from build123d import *

# Parameters (mm, degrees)
BOSS_EXTRUDE1_DEPTH = 6.35
SKETCH2_W           = 20
SKETCH2_H           = 6.35
CUT_EXTRUDE1_DEPTH  = 172.94569637
SKETCH4_W           = 6.35
SKETCH4_H           = 15
CUT_EXTRUDE2_DEPTH  = 172.94569637
FILLET1_R           = 2


with BuildPart() as part:
    # Sketch1 → Boss-Extrude1 (new body)
    with BuildSketch(Plane(origin=(0, 0, 0), x_dir=(1, 0, 0), z_dir=(0, 1, 0))):
        Polygon((-170, 0), (-170, 20), (0, 20), (7, 20), (7, -25), (0, -25), (-170, -25), align=None)
    extrude(amount=BOSS_EXTRUDE1_DEPTH)

    # Sketch2 → Cut-Extrude1 (cut, through all)
    with BuildSketch(Plane(origin=(0, 6.35, 0), x_dir=(1, 0, 0), z_dir=(0, 1, 0))):
        with Locations((-110, -16.825)):
            Rectangle(SKETCH2_W, SKETCH2_H)
        with Locations((-155, -16.825)):
            Rectangle(SKETCH2_W, SKETCH2_H)
        with Locations((-65, -16.825)):
            Rectangle(SKETCH2_W, SKETCH2_H)
        with Locations((-20, -16.825)):
            Rectangle(SKETCH2_W, SKETCH2_H)
        with Locations((-110, -3.175)):
            Rectangle(SKETCH2_W, SKETCH2_H)
        with Locations((-155, -3.175)):
            Rectangle(SKETCH2_W, SKETCH2_H)
        with Locations((-65, -3.175)):
            Rectangle(SKETCH2_W, SKETCH2_H)
        with Locations((-20, -3.175)):
            Rectangle(SKETCH2_W, SKETCH2_H)
    extrude(amount=-CUT_EXTRUDE1_DEPTH, mode=Mode.SUBTRACT)

    # Sketch4 → Cut-Extrude2 (cut, through all)
    with BuildSketch(Plane(origin=(0, 6.35, 0), x_dir=(1, 0, 0), z_dir=(0, 1, 0))):
        with Locations((0, -12.5)):
            Rectangle(SKETCH4_W, SKETCH4_H)
        with Locations((0, 7.5)):
            Rectangle(SKETCH4_W, SKETCH4_H)
    extrude(amount=-CUT_EXTRUDE2_DEPTH, mode=Mode.SUBTRACT)

    # Fillet1
    fillet1_edges = [part.edges().sort_by_distance(p)[0] for p in [
        (7, 3.175, -20),
        (7, 3.175, 25),
        (-170, 3.175, 25),
        (-170, 3.175, -20),
    ]]
    fillet(fillet1_edges, radius=FILLET1_R)


solid = part.part
Model file for the job. Use its own axes, mm. Give positions to 0.01 mm unless a question says otherwise; leave off trailing zeros. Order: outer loops, then holes, each group sorted by start corner. A loop starts at its lowest first (then second) coordinate and runs counter-clockwise, first axis right, second up. Notation, with made-up numbers: M -39.5,-36 L -21.5,-36 A6 cw -21.5,-28 Z; hole C -19.5,41 d3. An arc over 180 degrees is marked long. Put each result on its own line as item: value. Start each with the question number.
(1) Band-saw the part on A-A on x = -101.5. Give the cut face in (y, z), then the cut area to 3 significant figures.
(2) Pull direction Z, two halves, no side cores. Call faces 1 (the face through (-80, 3, -20)), 2 (the face through (-170, 3, 2)), 3 (the face through (-20, 3, 20)): released by +Z, released by -Z, zero draft, split by the parting line, or undercut.
(3) Band-saw the part on B-B on z = 9.5. Give the cut face in (x, y) (3 decimals).
(4) Band-saw the part on C-C on y = 2.25. Count the separate pieces of the cut face and the enclosed holes in it, then the cut area to 3 significant figures.
(5) Drill centre lines: L1, parallel to Z at x = -73.5, y = 3.5; L2, parallel to X at y = 3.25, z = 5.5 (3 decimals); L3, parallel to X at y = 6, z = -8 (3 decimals). Where is each one in solid material? Low to high. Write a range as [from, to].
Results below:
1. outline: M 0,-20 L 6.35,-20 L 6.35,0 L 0,0 Z; M 0,6.35 L 6.35,6.35 L 6.35,13.65 L 0,13.65 Z; M 0,20 L 6.35,20 L 6.35,25 L 0,25 Z
1. area: 205 mm2
2. face 1: released by -Z
2. face 2: zero draft
2. face 3: undercut
3. outline: M -170,0 L -3.175,0 L -3.175,6.35 L -170,6.35 Z; M 3.175,0 L 7,0 L 7,6.35 L 3.175,6.35 Z
4. separate pieces: 1
4. enclosed holes: 10
4. area: 6,760 mm2
5. L1: z = [-20, 0], [6.35, 13.65], [20, 25]
5. L2: x = [-170, -165], [-145, -120], [-100, -75], [-55, -30], [-10, -3.175], [3.175, 7]
5. L3: x = [-170, -3.175], [3.175, 7]
